```python
from build123d import *

# Parameters (mm, degrees)
SKETCH_2_W          = 102
SKETCH_2_H          = 53
EXTRUDE_1_DEPTH     = 2
CUT_EXTRUDE_1_DEPTH = 2
SKETCH_4_R          = 2
CUT_EXTRUDE_2_DEPTH = 2
FILLET_1_R          = 1
SKETCH_5_R          = 2
CUT_EXTRUDE_3_DEPTH = 2
SKETCH_6_W          = 17
SKETCH_6_H          = 12
EXTRUDE_2_DEPTH     = 10
SKETCH_7_W          = 70.5
SKETCH_7_H          = 2.5
SKETCH_7_W_2        = 5
SKETCH_7_H_2        = 45.597878471
SKETCH_7_W_3        = 71.552945179
EXTRUDE_3_DEPTH     = 8
SKETCH_8_W          = 15
SKETCH_8_H          = 15
EXTRUDE_4_DEPTH     = 1
SKETCH_9_W          = 1.65475178
SKETCH_9_H          = 2.5
CUT_EXTRUDE_4_DEPTH = 8
SKETCH_10_W         = 15
SKETCH_10_H         = 8.5
EXTRUDE_5_DEPTH     = 10
CUT_EXTRUDE_5_DEPTH = 10
SKETCH_12_R         = 3
SKETCH_12_R_2       = 0.5
CUT_EXTRUDE_6_DEPTH = 11
SKETCH_13_W         = 3
SKETCH_13_H         = 4
CUT_EXTRUDE_7_DEPTH = 11


with BuildPart() as part:
    # 草图2 → 凸台-拉伸1 (new body)
    with BuildSketch(Plane.XY):
        Rectangle(SKETCH_2_W, SKETCH_2_H)
    extrude(amount=EXTRUDE_1_DEPTH)

    # 草图3 → 切除-拉伸1 (cut)
    with BuildSketch(Plane.XY.offset(2)):
        Polygon((51, 11.5), (48, 14.5), (48, 24.5), (46, 26.5), (51, 26.5), align=None)
        Polygon((51, -21.5), (48, -25.5), (48, -26.5), (51, -26.5), align=None)
    extrude(amount=-CUT_EXTRUDE_1_DEPTH, mode=Mode.SUBTRACT)

    # 草图4 → 切除-拉伸2 (cut)
    with BuildSketch(Plane.XY.offset(2)):
        with Locations((46, -23.5)):
            Circle(SKETCH_4_R)
    extrude(amount=-CUT_EXTRUDE_2_DEPTH, mode=Mode.SUBTRACT)

    # 圆角1
    fillet_1_edges = [part.edges().sort_by_distance(p)[0] for p in [
        (48, -26.5, 1),
    ]]
    fillet(fillet_1_edges, radius=FILLET_1_R - 0.0001)  # a hair under: the kernel refuses the full size

    # 草图5 → 切除-拉伸3 (cut)
    with BuildSketch(Plane.XY.offset(2)):
        with Locations((39, 23.5)):
            Circle(SKETCH_5_R)
        with Locations((-36.5, 23.5)):
            Circle(SKETCH_5_R)
        with Locations(Location((-36.5, -23.5, 0), (0, 0, 180))):
            Circle(SKETCH_5_R)
    extrude(amount=-CUT_EXTRUDE_3_DEPTH, mode=Mode.SUBTRACT)

    # 草图6 → 凸台-拉伸2 (add)
    with BuildSketch(Plane.XY.offset(2)):
        with Locations((-49.5, 10.5)):
            Rectangle(SKETCH_6_W, SKETCH_6_H)
    extrude(amount=EXTRUDE_2_DEPTH)

    # 草图7 → 凸台-拉伸3 (add)
    with BuildSketch(Plane.XY.offset(2)):
        with Locations((1.25, 23.75)):
            Rectangle(SKETCH_7_W, SKETCH_7_H)
        with Locations((44.72661283, 2.201060764)):
            Rectangle(SKETCH_7_W_2, SKETCH_7_H_2)
        with Locations((6.72352741, -23.75)):
            Rectangle(SKETCH_7_W_3, SKETCH_7_H)
    extrude(amount=EXTRUDE_3_DEPTH)

    # 草图8 → 凸台-拉伸4 (add)
    with BuildSketch(Plane.XY.offset(2)):
        Rectangle(SKETCH_8_W, SKETCH_8_H)
    extrude(amount=EXTRUDE_4_DEPTH)

    # 草图9 → 切除-拉伸4 (cut)
    with BuildSketch(Plane.XY.offset(10)):
        with Locations((-6.746736472, -23.75)):
            Rectangle(SKETCH_9_W, SKETCH_9_H)
        with Locations((18.258401548, -23.75)):
            Rectangle(SKETCH_9_W, SKETCH_9_H)
    extrude(amount=-CUT_EXTRUDE_4_DEPTH, mode=Mode.SUBTRACT)

    # 草图10 → 凸台-拉伸5 (add)
    with BuildSketch(Plane.XY.offset(2)):
        with Locations((-46.5, -18.25)):
            Rectangle(SKETCH_10_W, SKETCH_10_H)
    extrude(amount=EXTRUDE_5_DEPTH)

    # 草图11 → 切除-拉伸5 (cut)
    with BuildSketch(Plane(origin=(-39, 0, 0), x_dir=(0, 0, -1), z_dir=(1, 0, 0))):
        with BuildLine():
            ThreePointArc((-7.75, -22.5), (-10.75520382, -21.25520382), (-12, -18.25))
            Line((-12, -18.25), (-12, -22.5))
            Line((-12, -22.5), (-7.75, -22.5))
        make_face()
        with BuildLine():
            Line((-7.75, -14), (-12, -14))
            Line((-12, -14), (-12, -18.25))
            ThreePointArc((-12, -18.25), (-10.75520382, -15.24479618), (-7.75, -14))
        make_face()
    extrude(amount=-CUT_EXTRUDE_5_DEPTH, mode=Mode.SUBTRACT)

    # 草图12 → 切除-拉伸6 (cut)
    with BuildSketch(Plane.ZY.offset(54)):
        with Locations((7.75, -18.25)):
            Circle(SKETCH_12_R)
        with Locations((7.75, -18.25)):
            Circle(SKETCH_12_R_2, mode=Mode.SUBTRACT)
    extrude(amount=-CUT_EXTRUDE_6_DEPTH, mode=Mode.SUBTRACT)

    # 草图13 → 切除-拉伸7 (cut)
    with BuildSketch(Plane.ZY.offset(58)):
        Polygon((11, 13.5), (9, 15.5), (3, 15.5), (3, 5.5), (9, 5.5), (11, 7.5), align=None)
        with Locations((7, 10.5)):
            Rectangle(SKETCH_13_W, SKETCH_13_H, mode=Mode.SUBTRACT)
    extrude(amount=-CUT_EXTRUDE_7_DEPTH, mode=Mode.SUBTRACT)


solid = part.part
```
Read the model definition and answer for the solid it produces. Units are mm, in the model's axes. A direction names the side the tool comes from. Round coordinates to 2 decimals unless told otherwise and drop trailing zeros. Write each loop counter-clockwise with the first axis right and the second up, starting at its lowest first coordinate (ties: lowest second). Pieces come first, ordered by that corner, then holes. Notation, with made-up numbers: (69, 60) - (120, 60) arc R22 cw to (120, 93) - close; hole circle Ø1 at (76.25, -10.75). An arc over 180 degrees is marked (long way). One line per item, written item: value.
Q1. Find section A-A (x = 39). Determine the outline of the cut face in (y, z).
The answers:
outline: (-26.5, 0) - (21.5, 0) - (21.5, 2) - (-22.5, 2) - (-22.5, 10) - (-25, 10) - (-25, 2) - (-26.5, 2) - close; (25.5, 0) - (26.5, 0) - (26.5, 2) - (25.5, 2) - close
Q2. Straight lines are drawn through the part: line 1 (Y direction, x = -49.5, z = 7.75); line 2 (Y direction, x = -36.5, z = 0.95); line 3 (Y direction, x = 10, z = 2.25). For each, find the intervals that lie inside material, in ascending order. Write a range as from..to.
The answers:
line 1: y = -22.5..-21.25, -18.75..-17.75, -15.25..-14, 4.5..5.5, 8.5..12.5, 15.5..16.5
line 2: y = -26.5..-25.5, -21.5..21.5, 25.5..26.5
line 3: y = -25..-22.5, 22.5..25
Q3. Find section B-B (x = -36.5). Determine the outline of the cut face in (y, z), and give its area (3 significant figures).
The answers:
outline: (-26.5, 0) - (-25.5, 0) - (-25.5, 2) - (-26.5, 2) - close; (-21.5, 0) - (21.5, 0) - (21.5, 2) - (-21.5, 2) - close; (25.5, 0) - (26.5, 0) - (26.5, 2) - (25.5, 2) - close
area: 90.0 mm2
Q4. Find section D-D (x = -11.5). Determine the outline of the cut face in (y, z).
The answers:
outline: (-26.5, 0) - (26.5, 0) - (26.5, 2) - (25, 2) - (25, 10) - (22.5, 10) - (22.5, 2) - (-22.5, 2) - (-22.5, 10) - (-25, 10) - (-25, 2) - (-26.5, 2) - close
Q5. Find section C-C (y = -23.5). Determine the outline of the cut face in (x, z), and give its area (3 significant figures).
The answers:
outline: (-51, 0) - (-38.5, 0) - (-38.5, 2) - (-51, 2) - close; (-34.5, 0) - (44, 0) - (44, 2) - (42.5, 2) - (42.5, 10) - (19.09, 10) - (19.09, 2) - (17.43, 2) - (17.43, 10) - (-5.92, 10) - (-5.92, 2) - (-7.57, 2) - (-7.57, 10) - (-29.05, 10) - (-29.05, 2) - (-34.5, 2) - close; (48, 0) - (49.5, 0) - (49.5, 2) - (48, 2) - close
area: 731 mm2
Q6. Each of these flat-tipped pins is pushed along its axis until it touches: P1, Ø2, axis at y = -23.5, z = 7, coming from the +X side; P2, Ø6.5, axis at x = 5, z = 8, coming from the -Y side; P3, Ø0.8, axis at y = -18.5, z = 7.5, coming from the -X side; P4, Ø2, axis at x = -19.5, y = 3, coming from the -Z side. Where does it stop, or does it pass through?
The answers:
P1: stops at x = 42.5
P2: stops at y = -25
P3: stops at x = -54
P4: stops at z = 0
Q7. For a pull along Z with two mould halves and no side action, classify faces 5 (the flat face through (-53, 8.5, 7)), 6 (the flat face through (-3, 26.5, 1)), 7 (the flat face through (-55, 11, 2)) as pulls with the +Z half, pulls with the -Z half, needs draft (parallel to the pull), parting line crosses it, or undercut.
The answers:
face 5: undercut
face 6: needs draft
face 7: pulls with the -Z half
Q8. Which of the six approach directions +Z, -Z, +X, -X, +Y, -Y give full straight-line access (tool end or side, diameter ignored) to faces 1 (the flat face through (45, 25, 6)), 2 (the flat face through (-52.6, 14.5, 10)), 3 (the flat face through (-41, 10, 7)), 4 (the flat face through (31, -22.5, 6))?
The answers:
face 1: +Z, +X, -X, +Y
face 2: -X
face 3: +Z, +Y
face 4: +Z, +X
